Autodesk Inventor part; units mm, degrees
ref_plane "YZ Plane" through (0, 0, 0) normal (1, 0, 0) x (0, 1, 0)
ref_plane "XZ Plane" through (0, 0, 0) normal (0, 1, 0) x (-1, 0, 0)
ref_plane "XY Plane" through (0, 0, 0) normal (0, 0, 1) x (1, 0, 0)
sketch "Эскиз1" plane through (0, 0, 0) normal (0, 0, 1) x (1, 0, 0)
  circle A0 centre (0, 0) radius 4.05
  line L0 (-6.05, -6.05) -> (6.05, -6.05)
  line L1 (6.05, -6.05) -> (6.05, 6.05)
  line L2 (6.05, 6.05) -> (-6.05, 6.05)
  line L3 (-6.05, 6.05) -> (-6.05, -6.05)
  line L4 (-6.05, -6.05) -> (6.05, 6.05) construction
  line L5 (6.05, -6.05) -> (-6.05, 6.05) construction
  line L6 (0, 4.05) -> (0, 6.05)
  line L7 (-4.05, 0) -> (-6.05, 0)
  line L8 (-15.15, -1.05) -> (0, -1.05)
  line L9 (0, -1.05) -> (0, -3.05)
  line L10 (0, -3.05) -> (-15.15, -3.05)
  line L11 (-15.15, -3.05) -> (-15.15, -1.05)
  line L12 (-4.05, 0) -> (4.05, 0)
  line L13 (4.05, 0) -> (4.05, -3.05)
  line L14 (4.05, -3.05) -> (-4.05, -3.05)
  line L15 (-4.05, -3.05) -> (-4.05, 0)
  line L16 (4.05, -3.05) -> (6.05, -3.05)
  line L17 (6.05, -3.05) -> (6.05, 0)
  line L18 (6.05, 0) -> (4.05, 0)
  line L19 (4.05, 0) -> (4.05, -3.05)
  point P0 (0, -2.05)
  point P1 (0, -6.05)
  point P2 (-6.05, -1.05)
  point P3 (-2.6646, -3.05)
  point P4 (-4.05, -3.05)
  point P5 (2.6646, -3.05)
  point P6 (-6.05, -3.05)
  point P7 (-4.05, -1.05)
  point P8 (-3.9115, -1.05)
  point P9 (-2.6646, -3.05)
  dimension "d0" = 8.1
  dimension "d1" = 2
  dimension "d2" = 2
  dimension "d3" = 9.1
  dimension "d4" = 2
  dimension "d5" = 3
extrude "Выдавливание1" add sketch "Эскиз1" along normal blind 1.7 contours A0 L7 L3 L2 L6 | L15 L8 L3 L7 | L15 L10 L3 L8 | L3 L10 L11 L8
sketch "Эскиз2" plane through (0, 0, 1.7) normal (0, 0, 1) x (1, 0, 0)
  line L0 (-6.05, -1.05) -> (-15.15, -1.05)
  line L1 (-15.15, -1.05) -> (-15.15, -3.05)
  line L2 (-15.15, -3.05) -> (-4.05, -3.05)
  line L3 (-4.05, -3.05) -> (-4.05, 0)
  arc A0 (0, 4.05) -> (-4.05, 0) centre (0, 0) ccw
  line L4 (0, 4.05) -> (0, 6.05)
  line L5 (0, 6.05) -> (-6.05, 6.05)
  line L6 (-6.05, 6.05) -> (-6.05, -1.05)
  line L7 (0, 4.05) -> (-4.05, 4.05)
  line L8 (-4.05, 4.05) -> (-4.05, -3.05)
  line L9 (-4.05, -3.05) -> (0, -3.05)
  line L10 (0, -3.05) -> (0, 4.05)
extrude "Выдавливание2" add sketch "Эскиз2" along normal blind 3
mirror "Зеркальное отражение1" about plane through (-9.6, -2.05, 0) normal (0, 0, -1)
sketch "Эскиз4" plane through (-15.15, -1.05, 4.7) normal (0, 1, 0) x (1, 0, 0)
  line L0 (0, 9.4) -> (0, 0)
  line L1 (0, 4.7) -> (9.1, 4.7)
  line L2 (9.1, 9.4) -> (9.1, 0)
  point P0 (15.15, 4.7)
  point P1 (4.55, 4.7)
hole "Отверстие2" at (-10.6, -1.05, 0) direction (0, -1, 0) diameter 3.2 end through all
mirror "Зеркальное отражение2" about plane through (0, 4.05, 0) normal (1, 0, 0)
sketch "Эскиз3" plane through (0, 0, 4.7) normal (0, 0, 1) x (1, 0, 0)
  arc A0 (2.6646, -3.05) -> (4.05, 0) centre (0, 0) ccw
  arc A1 (2.6646, -3.05) -> (4.05, 0) centre (0, 0) ccw
hole "Отверстие1" at (0, 0, 4.7) direction (0, 0, -1) diameter 5 end through all
fillet "Сопряжение1" radius 6.05 2 edges at (-6.05, 6.05, 0) (6.05, 6.05, 0)
sketch "Эскиз7" plane through (-15.15, -3.05, -4.7) normal (0, -1, 0) x (1, 0, 0)
  line L0 (30.3, 0) -> (0, 0)
  line L1 (0, 9.4) -> (30.3, 9.4)
  line L2 (12.65, 9.4) -> (17.65, 9.4)
  line L3 (15.15, 9.4) -> (15.15, 0)
  line L4 (28.3, 2) -> (2, 2)
  line L5 (2, 2) -> (2, 7.4)
  line L6 (2, 7.4) -> (28.3, 7.4)
  line L7 (28.3, 7.4) -> (28.3, 2)
  line L8 (28.3, 2) -> (2, 7.4) construction
  line L9 (2, 2) -> (28.3, 7.4) construction
  line L10 (0, 9.4) -> (0, 0)
  line L11 (30.3, 9.4) -> (30.3, 0)
  point P0 (15.15, 4.7)
  dimension "d29" = 2
  dimension "d30" = 2
extrude "Выдавливание4" add sketch "Эскиз7" along normal blind 7.75 contours L0 L3 L4 L7 L6 L1 L11 | L0 L10 L1 L3 L6 L5 L4
fillet "Сопряжение2" radius 4.7 4 edges at (15.15, -5.925, -4.7) (15.15, -5.925, 4.7) (-15.15, -5.925, -4.7) (-15.15, -5.925, 4.7)
fillet "Сопряжение3" radius 2.7 4 edges at (13.15, -6.925, -2.7) (13.15, -6.925, 2.7) (-13.15, -6.925, 2.7) (-13.15, -6.925, -2.7)
properties part number "Крышка стойки подшипника 3мм"
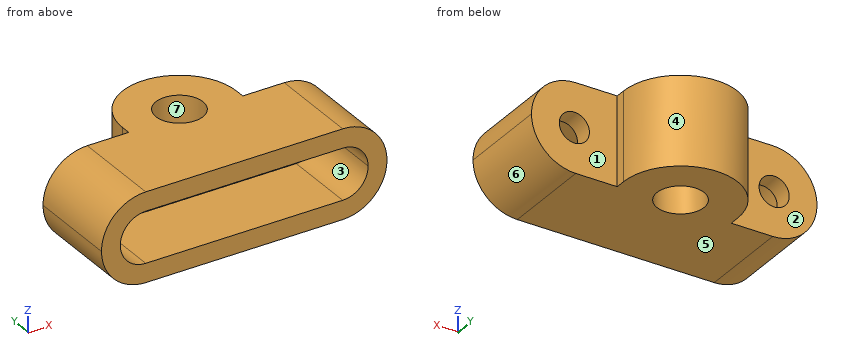
Build history of the part. All positions in model axes, mm. Face numbers are marked on the shaded views. A direction names the side the tool comes from. Coordinates: 2 decimals unless noted, no trailing zeros. Write each loop counter-clockwise with the first axis right and the second up, starting at its lowest first coordinate (ties: lowest second). Pieces come first, ordered by that corner, then holes.
1. Band-saw the part on C-C, the plane z = 1. Give the cut face in (x, y).
Answer block:
outline: (-15.04, -10.8) - (-12.96, -10.8) - (-12.96, -3.05) - (-11.85, -3.05) - (-11.85, -1.05) - (-15.04, -1.05) - close; (-9.35, -3.05) - (-4.05, -3.05) - (-4.05, 0) arc R4.05 cw to (4.05, 0) - (4.05, -3.05) - (9.35, -3.05) - (9.35, -1.05) - (6.05, -1.05) - (6.05, 0) arc R6.05 ccw to (-6.05, 0) - (-6.05, -1.05) - (-9.35, -1.05) - close; (11.85, -3.05) - (12.96, -3.05) - (12.96, -10.8) - (15.04, -10.8) - (15.04, -1.05) - (11.85, -1.05) - close
2. Band-saw the part on D-D, the plane y = 0.5. Give the cut face in (x, z), and give its area (3 significant figures).
Answer block:
outline: (-6.03, -4.7) - (-2.45, -4.7) - (-2.45, -1.7) - (-4.02, -1.7) - (-4.02, 1.7) - (-2.45, 1.7) - (-2.45, 4.7) - (-6.03, 4.7) - close; (2.45, -4.7) - (6.03, -4.7) - (6.03, 4.7) - (2.45, 4.7) - (2.45, 1.7) - (4.02, 1.7) - (4.02, -1.7) - (2.45, -1.7) - close
area: 56.6 mm2
3. 3-axis set-ups, long thin cutter, end or side, ignore diameter. For the marked faces 1, 2 and 3: which of +Z, -Z, +X, -X, +Y, -Y reach the whole face in a straight line?
Answer block:
face 1: +Z, -Z, +X, +Y
face 2: +Z, -Z, -X, +Y
face 3: -Y
4. Band-saw the part on A-A, the plane x = 0. Give the cut face in (y, z).
Answer block:
outline: (-10.8, -4.7) - (-2.5, -4.7) - (-2.5, -1.7) - (-3.05, -1.7) - (-3.05, -2.7) - (-10.8, -2.7) - close; (-10.8, 2.7) - (-3.05, 2.7) - (-3.05, 1.7) - (-2.5, 1.7) - (-2.5, 4.7) - (-10.8, 4.7) - close; (2.5, -4.7) - (6.05, -4.7) - (6.05, 4.7) - (2.5, 4.7) - (2.5, 1.7) - (4.05, 1.7) - (4.05, -1.7) - (2.5, -1.7) - close
5. Pull direction X, two halves, no side cores. Call the marked faces 4, 5, 6 and 7: released by +X, released by -X, zero draft, split by the parting line, or undercut.
Answer block:
face 4: split by the parting line
face 5: zero draft
face 6: released by +X
face 7: undercut
6. Drop flat-ended pins along their axis: pin 1 (5 mm diameter, centred on x = 10.6, z = 0, fed in from +Y); pin 2 (0.5 mm diameter, centred on y = -0.5, z = -2, fed in from +X); pin 3 (1 mm diameter, centred on x = 10, z = 1.5, fed in from -Y). Give the stop position or say it passes through.
Answer block:
pin 1: stops at y = -1.05
pin 2: stops at x = 6.05
pin 3: stops at y = -3.05
7. Drill centre lines: probe 1 along X at (y, z) = (-2.3, 0); probe 2 along X at (y, z) = (0, -2.35); probe 3 along Z at (x, y) = (-6.5, -6). Where is each one in solid material? Low to high.
Answer block:
probe 1: x = -15.15 to -12.2, -9 to -4.05, 4.05 to 9, 12.2 to 15.15
probe 2: x = -6.05 to -2.5, 2.5 to 6.05
probe 3: z = -4.7 to -2.7, 2.7 to 4.7
